Source: three-view drawing plus pictorial views. Frame: mm from the lowest corner of the part. Coordinates: 2 decimals unless noted, no trailing zeros. Order: outer loops, then holes, each group sorted by start corner. A loop starts at its lowest first (then second) coordinate and runs counter-clockwise, first axis right, second up. Notation, with made-up numbers: M 55,86.25 L 101,86.25 A25 cw 101,105.25 Z; hole C 67,16.5 d11. An arc over 180 degrees is marked long. Write item = value, one per line. Start each with the question number.
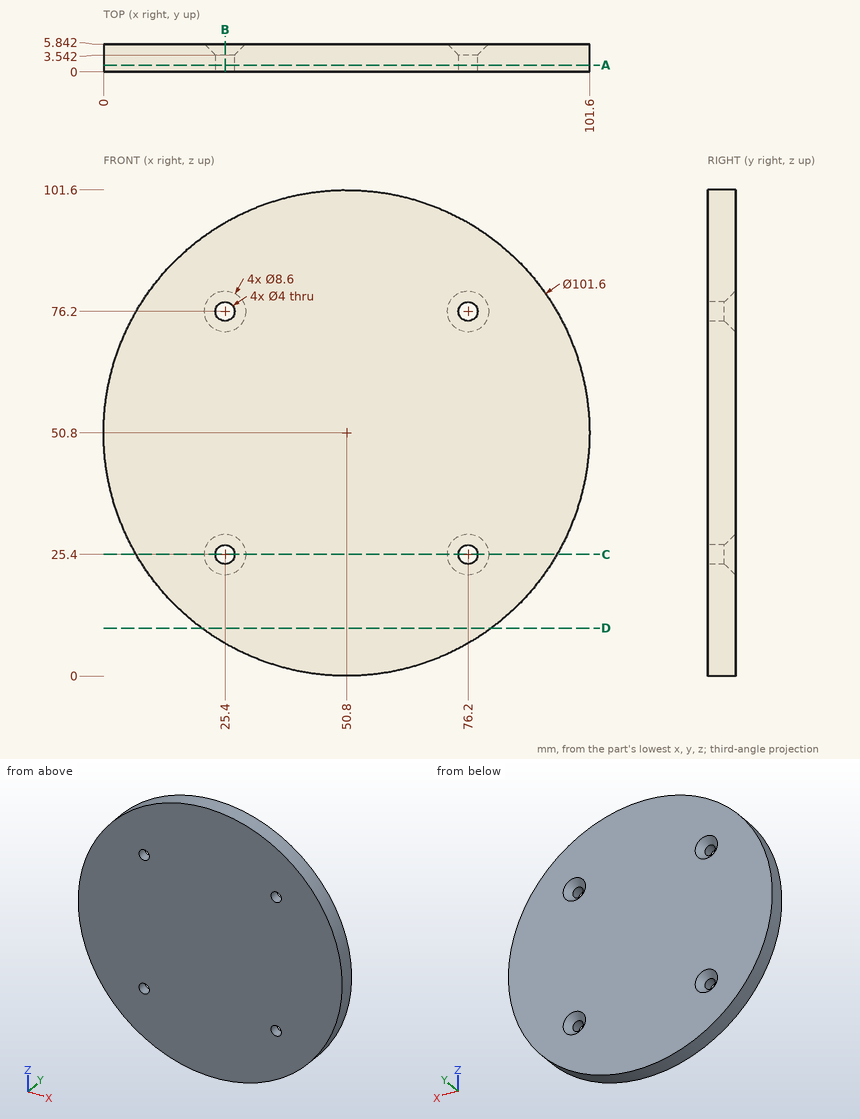
Item 1: Section query C-C on z = 25.4. Output: boundary loops of the cut face in (x, y), and give its area (3 significant figures).
Item 2: Section query B-B on x = 25.4. Output: boundary loops of the cut face in (y, z).
Item 3: Material intervals for probe 1 along Z at (x, y) = (26.5, 3.15); probe 2 along X at (y, z) = (2.4, 76.2); probe 3 along X at (y, z) = (1.7, 26), sorted ascending. Write a range as [from, to].
Item 4: Section query D-D on z = 10. Output: boundary loops of the cut face in (x, y).
Item 5: First-contact query: pin 1 (3 mm diameter, centred on y = 4.5, z = 86.5, fed in from +X); pin 2 (3 mm diameter, centred on x = 26.5, y = 4.5, fed in from +Z); pin 3 (1 mm diameter, centred on x = 46, y = 3.5, fed in from -Z). Flat tips, straight axial feed; report the tip coordinate or a pass-through.
Item 6: Section query A-A on y = 1.4. Output: boundary loops of the cut face in (x, z).
Ans:
q1.outline = M 6.81,0 L 23.4,0 L 23.4,3.54 L 21.1,5.84 L 6.81,5.84 Z; M 27.4,0 L 74.2,0 L 74.2,3.54 L 71.9,5.84 L 29.7,5.84 L 27.4,3.54 Z; M 78.2,0 L 94.79,0 L 94.79,5.84 L 80.5,5.84 L 78.2,3.54 Z
q1.area = 457 mm^2
q2.outline = M 0,6.81 L 5.84,6.81 L 5.84,21.1 L 3.54,23.4 L 0,23.4 Z; M 0,27.4 L 3.54,27.4 L 5.84,29.7 L 5.84,71.9 L 3.54,74.2 L 0,74.2 Z; M 0,78.2 L 3.54,78.2 L 5.84,80.5 L 5.84,94.79 L 0,94.79 Z
q3.probe_1 = [6.19, 23.73], [27.07, 74.53], [77.87, 95.41]
q3.probe_2 = [6.81, 23.4], [27.4, 74.2], [78.2, 94.79]
q3.probe_3 = [6.46, 23.49], [27.31, 74.29], [78.11, 95.14]
q4.outline = M 20.53,0 L 81.07,0 L 81.07,5.84 L 20.53,5.84 Z
q5.pin_1 = 88.36
q5.pin_2 = 96.2
q5.pin_3 = 0.18
q6.outline = C 50.8,50.8 d101.6; hole C 25.4,25.4 d4; hole C 25.4,76.2 d4; hole C 76.2,25.4 d4; hole C 76.2,76.2 d4
